Geometry: final body of the model. Coordinates: model frame, mm. Face numbers are marked on the shaded views. Give positions to 0.01 mm unless a question says otherwise; leave off trailing zeros. Write each loop counter-clockwise with the first axis right and the second up, starting at its lowest first coordinate (ties: lowest second). Pieces come first, ordered by that corner, then holes. Notation, with made-up numbers: M 22.5,16 L 65.5,16 A34 ccw 65.5,52 Z; hole C -6.75,50.5 d10. An arc over 180 degrees is marked long. Use a Markdown table: item, result. Add a question column.
1) Line query: line 1 (X direction, y = -3.95, z = 53) (3 decimals); line 2 (X direction, y = -1.7, z = -53); line 3 (X direction, y = -4, z = -42). Output: solid intervals per line, ascending.
2) Pin query (flat end, axial travel): pin 1 (1.5 mm diameter, centred on x = -5, z = -47, fed in from +Y); pin 2 (3 mm diameter, centred on x = -2, y = -4.5, fed in from +Z); pin 3 (5 mm diameter, centred on x = -7.5, z = -53, fed in from -Y); pin 4 (1.9 mm diameter, centred on x = -7.5, z = -53, fed in from +Y). Return the tip coordinate at first contact, or that it passes through.
3) Section A-A on z = -40. Return the cut outline in (x, y).
4) Section B-B on z = 53. Return the cut outline in (x, y) (3 decimals).
5) Draft query along X for the marked faces 1 and 2. Return one class per face: +X half, -X half, draft (parallel to the pull), parting line (faces both ways), or undercut.
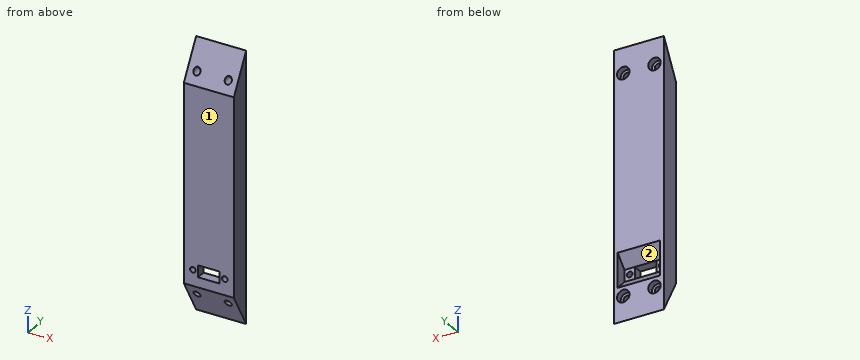
```python
from build123d import *

# Parameters (mm, degrees)
BOSS_EXTRUDE1_DEPTH     = 12
CUT_EXTRUDE1_DEPTH      = 67.850579653
CUT_EXTRUDE1_DEPTH_BACK = 5.5
SKETCH2_W               = 20.3
SKETCH2_H               = 5.7
SKETCH3_W               = 10.3
SKETCH3_H               = 5.7
SKETCH3_R               = 1.35
CUT_EXTRUDE2_DEPTH      = 5.5
CHAMFER1_SIZE           = 5.5
SKETCH4_R               = 1.625
CUT_EXTRUDE3_DEPTH      = 67.850579653
SKETCH5_R               = 3
CUT_EXTRUDE4_DEPTH      = 3


with BuildPart() as part:
    # Sketch1 → Boss-Extrude1 (new, symmetric)
    with BuildSketch(Plane(origin=(0, 0, 0), x_dir=(0, 0, -1), z_dir=(1, 0, 0))):
        Polygon((-65, 0), (65, 0), (47.679491924, -10), (-47.679491924, -10), align=None)
    extrude(amount=BOSS_EXTRUDE1_DEPTH, both=True)

    # Sketch2 → Cut-Extrude1 (cut, two sides: drawn at the far end of the back side and taken through both)
    with BuildSketch(Plane(origin=(0, 0, 0), x_dir=(1, 0, 0), z_dir=(0, 1, 0)).offset(-CUT_EXTRUDE1_DEPTH_BACK)):
        with Locations((0, 40)):
            Rectangle(SKETCH2_W, SKETCH2_H)
    extrude(amount=CUT_EXTRUDE1_DEPTH + CUT_EXTRUDE1_DEPTH_BACK, mode=Mode.SUBTRACT)

    # Sketch3 → Cut-Extrude2 (cut)
    with BuildSketch(Plane(origin=(0, -5.5, 0), x_dir=(1, 0, 0), z_dir=(0, 1, 0))):
        with Locations((0, 40)):
            Rectangle(SKETCH3_W, SKETCH3_H)
        with Locations(Location((-7.65, 40, 0), (0, 0, 270))):
            Circle(SKETCH3_R)
        with Locations(Location((7.65, 40, 0), (0, 0, 270))):
            Circle(SKETCH3_R)
    extrude(amount=-CUT_EXTRUDE2_DEPTH, mode=Mode.SUBTRACT)

    # Chamfer1
    chamfer1_edges = [part.edges().sort_by_distance(p)[0] for p in [
        (0, 0, -37.15),
        (0, 0, -42.85),
    ]]
    chamfer(chamfer1_edges, length=CHAMFER1_SIZE - 0.0001)  # a hair under: the kernel refuses the full size

    # Sketch4 → Cut-Extrude3 (cut, through all)
    with BuildSketch(Plane(origin=(0, 0, 0), x_dir=(1, 0, 0), z_dir=(0, 1, 0))):
        with Locations(Location((-7.5, 53, 0), (0, 0, 270))):
            Circle(SKETCH4_R)
        with Locations(Location((7.5, 53, 0), (0, 0, 270))):
            Circle(SKETCH4_R)
    cut_extrude3 = extrude(amount=-CUT_EXTRUDE3_DEPTH, mode=Mode.SUBTRACT)

    # Sketch5 → Cut-Extrude4 (cut)
    with BuildSketch(Plane(origin=(0, 0, 0), x_dir=(1, 0, 0), z_dir=(0, 1, 0))):
        with Locations(Location((-7.5, 53, 0), (0, 0, 270))):
            Circle(SKETCH5_R)
        with Locations(Location((7.5, 53, 0), (0, 0, 270))):
            Circle(SKETCH5_R)
    cut_extrude4 = extrude(amount=-CUT_EXTRUDE4_DEPTH, mode=Mode.SUBTRACT)

    # Mirror1: Cut-Extrude3, Cut-Extrude4 across plane
    add(cut_extrude3.mirror(Plane.XY), mode=Mode.SUBTRACT)
    add(cut_extrude4.mirror(Plane.XY), mode=Mode.SUBTRACT)


solid = part.part
```
Found:
| question | item | result |
|---|---|---|
| 1 | line 1 | -12 to -9.125, -5.875 to 5.875, 9.125 to 12 |
| 1 | line 2 | -12 to -10.5, -4.5 to 4.5, 10.5 to 12 |
| 1 | line 3 | -12 to -10.15, 10.15 to 12 |
| 2 | pin 1 | y = -0.6 |
| 2 | pin 2 | z = 59.8 |
| 2 | pin 3 | y = -8.37 |
| 2 | pin 4 | through |
| 3 | outline | M -12,-10 L -9,-10 L -9,-5.5 L -10.15,-5.5 L -10.15,0 L -12,0 Z; M -6.3,-10 L -5.15,-10 L -5.15,-5.5 L -6.3,-5.5 Z; M 5.15,-10 L 6.3,-10 L 6.3,-5.5 L 5.15,-5.5 Z; M 9,-10 L 12,-10 L 12,0 L 10.15,0 L 10.15,-5.5 L 9,-5.5 Z |
| 4 | outline | M -12,-6.928 L -9.125,-6.928 L -9.125,-3 L -10.5,-3 L -10.5,0 L -12,0 Z; M -5.875,-6.928 L 5.875,-6.928 L 5.875,-3 L 4.5,-3 L 4.5,0 L -4.5,0 L -4.5,-3 L -5.875,-3 Z; M 9.125,-6.928 L 12,-6.928 L 12,0 L 10.5,0 L 10.5,-3 L 9.125,-3 Z |
| 5 | face 1 | draft |
| 5 | face 2 | undercut |
